Source: CAD feature listing. Evaluate the final solid. Frame: model axes, mm. Give positions to 0.01 mm unless a question says otherwise; leave off trailing zeros. Loops run counter-clockwise (first coordinate to the right, second up) from the corner with the lowest first, then second, coordinate; pieces in that order, holes last.
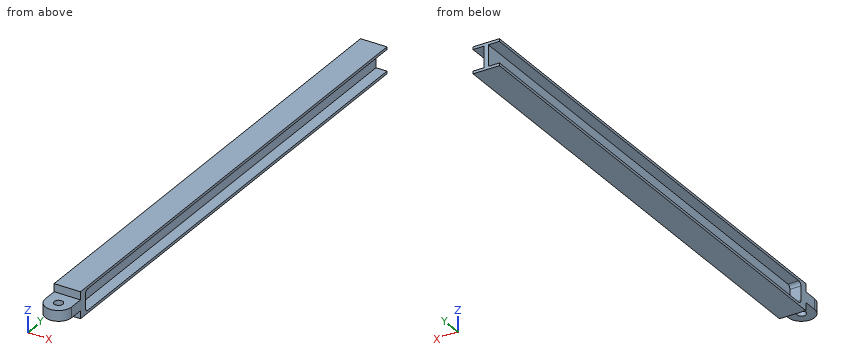
from build123d import *

# Parameters (mm, degrees)
EXTRUDE4_DEPTH     = 550
SKETCH4_W          = 30
SKETCH4_H          = 30
EXTRUDE5_DEPTH     = 40
SKETCH5_W          = 30
SKETCH5_H          = 9
CUT_EXTRUDE2_DEPTH = 31
SKETCH6_R          = 5
CUT_EXTRUDE3_DEPTH = 551.678899178
SKETCH7_OUTSIDE_W  = 150.304
SKETCH7_OUTSIDE_H  = 710.304
CUT_EXTRUDE4_DEPTH = 551.678899178
FILLET2_R          = 4
FILLET3_R          = 4


with BuildPart() as part:
    # Sketch1 → Extrude4 (new body)
    with BuildSketch(Plane(origin=(0, 0, 0), x_dir=(1, 0, 0), z_dir=(0, 1, 0))):
        Polygon((-12.5, 3), (17.5, 3), (17.5, 0), (5, 0), (5, -24), (17.5, -24), (17.5, -27), (-12.5, -27), (-12.5, -24), (0, -24), (0, 0), (-12.5, 0), align=None)
    extrude(amount=EXTRUDE4_DEPTH)

    # Sketch4 → Extrude5 (add)
    with BuildSketch(Plane.XZ):
        with Locations((2.5, 12)):
            Rectangle(SKETCH4_W, SKETCH4_H)
    extrude(amount=EXTRUDE5_DEPTH)

    # Sketch5 → Cut-Extrude2 (cut)
    with BuildSketch(Plane.XZ.offset(40)):
        with Locations((2.5, 1.5)):
            Rectangle(SKETCH5_W, SKETCH5_H)
        with Locations((2.5, 22.5)):
            Rectangle(SKETCH5_W, SKETCH5_H)
    extrude(amount=-CUT_EXTRUDE2_DEPTH, mode=Mode.SUBTRACT)

    # Sketch6 → Cut-Extrude3 (cut, through all)
    with BuildSketch(Plane.XY.offset(18)):
        with Locations((2.5, -25)):
            Circle(SKETCH6_R)
    extrude(amount=-CUT_EXTRUDE3_DEPTH, mode=Mode.SUBTRACT)

    # Sketch7 outside → Cut-Extrude4 (cut, through all)
    with BuildSketch(Plane.XY.offset(18)):
        with Locations((2.5, 255)):
            Rectangle(SKETCH7_OUTSIDE_W, SKETCH7_OUTSIDE_H)
        with BuildLine():
            Line((-12.5, 573.573250903), (17.5, 573.573250903))
            Line((17.5, 573.573250903), (17.5, -25))
            ThreePointArc((17.5, -25), (2.5, -40), (-12.5, -25))
            Line((-12.5, -25), (-12.5, 573.573250903))
        make_face(mode=Mode.SUBTRACT)
    extrude(amount=-CUT_EXTRUDE4_DEPTH, mode=Mode.SUBTRACT)

    # Fillet2
    fillet2_edges = [part.edges().sort_by_distance(p)[0] for p in [
        (11.25, 0, 24),
        (11.25, 0, 0),
    ]]
    fillet(fillet2_edges, radius=FILLET2_R)

    # Fillet3
    fillet3_edges = [part.edges().sort_by_distance(p)[0] for p in [
        (-6.25, 0, 0),
        (-6.25, 0, 24),
    ]]
    fillet(fillet3_edges, radius=FILLET3_R)


solid = part.part
1) Cut plane A-A (y = 288.5). Return loops of the section in (x, z), and give its area (3 significant figures).
Checks:
outline: (-12.5, -3) - (17.5, -3) - (17.5, 0) - (5, 0) - (5, 24) - (17.5, 24) - (17.5, 27) - (-12.5, 27) - (-12.5, 24) - (0, 24) - (0, 0) - (-12.5, 0) - close
area: 300 mm2
2) Ray query, probe 1 along Y at (x, z) = (2.5, 14.5); probe 2 along Z at (x, y) = (10, 169); probe 3 along Y at (x, z) = (9.25, 18.25). Return the intervals inside material, ascending.
Checks:
probe 1: y = -40 to -30, -20 to 550
probe 2: z = -3 to 0, 24 to 27
probe 3: y = -9 to 0
3) Contact query for flat-ended pins moving along their axis: P1, Ø4, axis at x = 14, z = 15, coming from the +Y side; P2, Ø5, axis at y = 117, z = 13.5, coming from the -X side; P3, Ø7, axis at x = 4.5, z = 2, coming from the -Y side; P4, Ø12, axis at y = 357.5, z = 20, coming from the +X side. Output: stop coordinate, or through.
Checks:
P1: stops at y = 0
P2: stops at x = 0
P3: stops at y = -9
P4: stops at x = 17.5
